Check sheet for the modelled part. Datum: model origin and axes. Units: mm. A direction names the side the tool comes from. Round coordinates to 2 decimals unless told otherwise and drop trailing zeros.
from build123d import *

# Parameters (mm, degrees)
F0_R     = 27
F0_R_2   = 22
F1_DEPTH = 15
F2_R     = 31
F2_R_2   = 27
F2_R_3   = 22
F3_DEPTH = 5
F4_W     = 1.5
F4_H     = 1
F6_SIZE2 = 1.49999
F6_SIZE  = 1.49999


# Not quite as in the source:
# - a fillet or chamfer is up to 0.001 mm smaller than in the source, because OpenCascade refuses the exact size


with BuildPart() as f1:
    # F0 (on Top) → F1 (new body)
    with BuildSketch(Plane.XY):
        Circle(F0_R)
        Circle(F0_R_2, mode=Mode.SUBTRACT)
    extrude(amount=F1_DEPTH)

    # F2 (on face) → F3 (join)
    with BuildSketch(Plane.XY.offset(15)):
        Circle(F2_R)
        Circle(F2_R_2, mode=Mode.SUBTRACT)
        Circle(F2_R_2)
        Circle(F2_R_3, mode=Mode.SUBTRACT)
        Circle(F2_R_3)
    extrude(amount=F3_DEPTH)

    # F4 (on Front) → F5 (revolve, cut)
    with BuildSketch(Plane.XZ):
        with Locations((-26.25, 2.5)):
            Rectangle(F4_W, F4_H)
        with Locations((-26.25, 7.5)):
            Rectangle(F4_W, F4_H)
        with Locations((-26.25, 12.5)):
            Rectangle(F4_W, F4_H)
    revolve(axis=Axis((0, 0, 9.1704530641), (0, 0, -1)), mode=Mode.SUBTRACT)

    # F6 (size 1.5 and 1.5 in the source; OpenCascade refuses exactly that, so slightly less here)
    f6_edges = [f1.edges().sort_by_distance(p)[0] for p in [
        (-27, 0, 3),
        (27, 0, 5),
        (-27, 0, 7),
        (-27, 0, 2),
        (-27, 0, 8),
        (27, 0, 10),
        (-27, 0, 12),
        (-27, 0, 13),
    ]]
    chamfer(f6_edges, length=F6_SIZE, length2=F6_SIZE2)


solid = f1.part
1. Set-up check for faces 5 (the flat face through (0, 0, 15)), 6 (the flat face through (-10, -20, 0)), 7 (the cylindrical face through (5.5, -24.9, 12.5)): record each of +Z, -Z, +X, -X, +Y, -Y from which the full face is reachable in a straight line by a thin tool's end or side.
2. Release check for a two-part mould opening along Z. For faces 1 (the cylindrical face through (5.5, -24.9, 2.5)), 2 (the cylindrical face through (-5.85, -26.36, 0.25)), 3 (the flat face through (2, 28, 15)), 4 (the cylindrical face through (5.5, -24.9, 7.5)) record: released by +Z, released by -Z, zero draft, split by the parting line, or undercut.
3. Go/stop test with flat-tipped pins: pin 1 (12 mm diameter, centred on x = 12.5, y = 8.5, fed in from -Z); pin 2 (3 mm diameter, centred on y = -10.5, z = 5.5, fed in from +X); pin 3 (10 mm diameter, centred on x = 22.5, z = 16, fed in from -Y); pin 4 (22 mm diameter, centred on x = 1, y = -11, fed in from -Z). Record where each tip stops, or that it passes through.
4. Scan lines: line 1 along Z through (x, y) = (-8, 8); line 2 along Y through (x, z) = (0, 8.75); line 3 along Y through (x, z) = (0, 5). Record each from-to range of solid material in increasing order.
Computed values:
1. face 5: -Z
1. face 6: -Z, +X, -X, +Y, -Y
1. face 7: none
2. face 1: undercut
2. face 2: zero draft
2. face 3: released by -Z
2. face 4: undercut
3. pin 1: stops at z = 15
3. pin 2: stops at x = 25.46
3. pin 3: stops at y = -25.59
3. pin 4: stops at z = 0
4. line 1: z = 15 to 20
4. line 2: y = -26.25 to -22, 22 to 26.25
4. line 3: y = -27 to -22, 22 to 27
